Here's how the part is built. I have some questions about the finished solid (model axes, mm). A direction names the side the tool comes from. Round coordinates to 2 decimals unless told otherwise and drop trailing zeros. Write each loop counter-clockwise with the first axis right and the second up, starting at its lowest first coordinate (ties: lowest second). Pieces come first, ordered by that corner, then holes. Notation, with made-up numbers: (-38.75, 77.25) -> (15.25, 77.25) arc R16 ccw to (15.25, 99.25) -> close; hole circle Ø2 at (54, -14). An arc over 180 degrees is marked (long way). Answer in a Markdown table with one row per item.
from build123d import *

# Parameters (mm, degrees)
CROQUIS1_W                 = 56.1
CROQUIS1_H                 = 26.6
CROQUIS1_R                 = 2.1
CROQUIS1_W_2               = 40.9
CROQUIS1_H_2               = 20.6
SALIENTE_EXTRUIR1_DEPTH    = 8
CROQUIS2_W                 = 50.6
CROQUIS2_H                 = 26.6
SALIENTE_EXTRUIR2_DEPTH    = 8
CROQUIS3_W                 = 60.73602496
CROQUIS3_H                 = 26.6
SALIENTE_EXTRUIR3_DEPTH    = 8
CROQUIS4_R                 = 11.25
CORTAR_EXTRUIR1_DEPTH      = 5.5
CROQUIS5_R                 = 5.1
CORTAR_EXTRUIR2_DEPTH      = 62.563808362
CROQUIS6_R                 = 12.05
CROQUIS6_R_2               = 11.05
SALIENTE_EXTRUIR4_DEPTH    = 0.3
CHAFL_N1_SIZE              = 0.3
REDONDEO1_R                = 0.15
CHAFL_N2_SIZE              = 5
CORTAR_EXTRUIR5_REACH      = 65.536
CROQUIS11_W                = 30.047801794
CROQUIS11_H                = 26.6
CROQUIS12_R                = 1.45
CORTAR_EXTRUIR6_DEPTH      = 62.821699265
CHAFL_N8_SIZE              = 3
CHAFL_N9_SIZE              = 1
CHAFL_N10_SIZE             = 1.5
SALIENTE_EXTRUIR7_DEPTH    = 3
REDONDEO3_R                = 5
CROQUIS14_R                = 1.45
CORTAR_EXTRUIR7_DEPTH      = 70.085008007
CORTAR_EXTRUIR8_DEPTH      = 70.085008007
CORTAR_EXTRUIR8_DEPTH_BACK = 70.085008007
CROQUIS15_R                = 1.45


with BuildPart() as part:
    # Croquis1 → Saliente-Extruir1 (new body)
    with BuildSketch(Plane.XY):
        Rectangle(CROQUIS1_W, CROQUIS1_H)
        with Locations((24.250000128, -5)):
            Circle(CROQUIS1_R, mode=Mode.SUBTRACT)
        with Locations((24.250000128, 5)):
            Circle(CROQUIS1_R, mode=Mode.SUBTRACT)
        with Locations((-24.249999872, -5)):
            Circle(CROQUIS1_R, mode=Mode.SUBTRACT)
        with Locations((-24.249999872, 5)):
            Circle(CROQUIS1_R, mode=Mode.SUBTRACT)
        Rectangle(CROQUIS1_W_2, CROQUIS1_H_2, mode=Mode.SUBTRACT)
    extrude(amount=SALIENTE_EXTRUIR1_DEPTH)

    # Croquis2 → Saliente-Extruir2 (add)
    with BuildSketch(Plane(origin=(28.05, 0, 0), x_dir=(0, 0, -1), z_dir=(1, 0, 0))):
        with Locations((17.3, 0)):
            Rectangle(CROQUIS2_W, CROQUIS2_H)
    extrude(amount=SALIENTE_EXTRUIR2_DEPTH)

    # Croquis3 → Saliente-Extruir3 (add)
    with BuildSketch(Plane(origin=(0, 0, -42.6), x_dir=(-1, 0, 0), z_dir=(0, 0, -1))):
        with Locations((-5.68198752, 0)):
            Rectangle(CROQUIS3_W, CROQUIS3_H)
    extrude(amount=-SALIENTE_EXTRUIR3_DEPTH)

    # Croquis4 → Cortar-Extruir1 (cut)
    with BuildSketch(Plane.XY.offset(-34.6)):
        with Locations((-10.53602496, 0)):
            Circle(CROQUIS4_R)
    extrude(amount=-CORTAR_EXTRUIR1_DEPTH, mode=Mode.SUBTRACT)

    # Croquis5 → Cortar-Extruir2 (cut, through all)
    with BuildSketch(Plane.XY.offset(-40.1)):
        with Locations((-10.53602496, 0)):
            Circle(CROQUIS5_R)
    extrude(amount=-CORTAR_EXTRUIR2_DEPTH, mode=Mode.SUBTRACT)

    # Croquis6 → Saliente-Extruir4 (add)
    with BuildSketch(Plane.XY.offset(-34.6)):
        with Locations((-10.53602496, 0)):
            Circle(CROQUIS6_R)
        with Locations((-10.53602496, 0)):
            Circle(CROQUIS6_R_2, mode=Mode.SUBTRACT)
    extrude(amount=SALIENTE_EXTRUIR4_DEPTH)

    # Chaflán1
    chafl_n1_edges = [part.edges().sort_by_distance(p)[0] for p in [
        (-22.58602496, 0, -34.6),
    ]]
    chamfer(chafl_n1_edges, length=CHAFL_N1_SIZE - 0.0001)  # a hair under: the kernel refuses the full size

    # Redondeo1
    redondeo1_edges = [part.edges().sort_by_distance(p)[0] for p in [
        (-21.58602496, 0, -34.6),
        (-21.58602496, 0, -34.3),
    ]]
    fillet(redondeo1_edges, radius=REDONDEO1_R - 0.0001)  # a hair under: the kernel refuses the full size

    # Chaflán2
    chafl_n2_edges = [part.edges().sort_by_distance(p)[0] for p in [
        (-24.68602496, -13.3, -38.6),
        (-24.68602496, 13.3, -38.6),
    ]]
    chamfer(chafl_n2_edges, length=CHAFL_N2_SIZE)

    # Croquis11 → Cortar-Extruir5 (cut, up to next)
    with BuildSketch(Plane.XY.offset(8), mode=Mode.PRIVATE) as cortar_extruir5_sk1:
        with Locations((-15.023900897, 0)):
            Rectangle(CROQUIS11_W, CROQUIS11_H)
    cortar_extruir5_tool1 = extrude(cortar_extruir5_sk1.sketch, amount=-CORTAR_EXTRUIR5_REACH, mode=Mode.PRIVATE) & part.part
    add(cortar_extruir5_tool1.solids().sort_by_distance((-15.023901, 0, 8))[0], mode=Mode.SUBTRACT)

    # Croquis12 → Cortar-Extruir6 (cut, through all)
    with BuildSketch(Plane(origin=(0, -13.3, 0), x_dir=(-1, 0, 0), z_dir=(0, -1, 0))):
        with Locations(Location((-4.5, -4, 0), (0, 0, 90))):
            Circle(CROQUIS12_R)
    extrude(amount=-CORTAR_EXTRUIR6_DEPTH, mode=Mode.SUBTRACT)

    # Chaflán8
    chafl_n8_edges = [part.edges().sort_by_distance(p)[0] for p in [
        (-24.68602496, 0, -42.6),
        (-22.18602496, -10.8, -42.6),
        (-22.18602496, 10.8, -42.6),
        (8.18198752, -13.3, -42.6),
        (8.18198752, 13.3, -42.6),
        (36.05, 0, -42.6),
    ]]
    chamfer(chafl_n8_edges, length=CHAFL_N8_SIZE)

    # Chaflán9
    chafl_n9_edges = [part.edges().sort_by_distance(p)[0] for p in [
        (-15.63602496, 0, -42.6),
    ]]
    chamfer(chafl_n9_edges, length=CHAFL_N9_SIZE)

    # Chaflán10
    chafl_n10_edges = [part.edges().sort_by_distance(p)[0] for p in [
        (18.025, -13.3, 8),
        (36.05, 0, 8),
        (18.025, 13.3, 8),
    ]]
    chamfer(chafl_n10_edges, length=CHAFL_N10_SIZE)

    # Croquis13 → Saliente-Extruir7 (add)
    with BuildSketch(Plane(origin=(0, 13.3, 0), x_dir=(1, 0, 0), z_dir=(0, 1, 0))):
        with BuildLine():
            Line((28.05, 8.144334064), (28.05, 0))
            Line((28.05, 0), (9, 0))
            add(Edge.make_bspline(
                [(9, 0), (24.941361066, 0.053648998), (28.05, 8.144334064)],
                knots=[0, 0, 0, 0.673633708, 0.673633708, 0.673633708], degree=2))
        make_face()
    saliente_extruir7 = extrude(amount=-SALIENTE_EXTRUIR7_DEPTH)

    # Simetría7: Saliente-Extruir7 across plane
    add(saliente_extruir7.mirror(Plane.ZX))

    # Redondeo3
    redondeo3_edges = [part.edges().sort_by_distance(p)[0] for p in [
        (28.05, 0, -34.6),
    ]]
    fillet(redondeo3_edges, radius=REDONDEO3_R)

    # Croquis14 → Cortar-Extruir7 (cut, through all)
    with BuildSketch(Plane.ZY.offset(-28.05)):
        with Locations((-15.372167032, -8.3)):
            Circle(CROQUIS14_R)
        with Locations((-25.372167032, -8.3)):
            Circle(CROQUIS14_R)
    cortar_extruir7 = extrude(amount=-CORTAR_EXTRUIR7_DEPTH, mode=Mode.SUBTRACT)

    # Simetría8: Cortar-Extruir7 across plane
    add(cortar_extruir7.mirror(Plane.ZX), mode=Mode.SUBTRACT)

    # Croquis15 → Cortar-Extruir8 (cut, two sides: drawn at the far end of the back side and taken through both)
    with BuildSketch(Plane.ZY.offset(-28.05).offset(-CORTAR_EXTRUIR8_DEPTH_BACK)):
        with Locations((-20.372167032, 0)):
            Circle(CROQUIS15_R)
        with Locations((-30.372167032, 0)):
            Circle(CROQUIS15_R)
    extrude(amount=CORTAR_EXTRUIR8_DEPTH + CORTAR_EXTRUIR8_DEPTH_BACK, mode=Mode.SUBTRACT)


solid = part.part
1) I need wall thicknesses on line 1 (Z direction, x = 31, y = 8.3); line 2 (Y direction, x = 24, z = 2); line 3 (X direction, y = -11.8, z = 4). Which ranges of each line are inside material? Lowest first, please. Write a range as [from, to].
Response:
| item | result |
|---|---|
| line 1 | z = [-42.6, -26.82], [-23.92, -16.82], [-13.92, 8] |
| line 2 | y = [-13.3, -7.09], [-2.91, 2.91], [7.09, 13.3] |
| line 3 | x = [0, 3.05], [5.95, 36.05] |
2) We'd pull the mould along Z, two halves only. Please class faces 1 (the face through (0, -12, 4)), 2 (the face through (8.6, -11.8, -41.1)), 3 (the face through (4, 12, 0)), 4 (the face through (31.99, 7.08, -14.59)): +Z half, -Z half, draft (parallel to the pull), parting line (faces both ways), or undercut.
Response:
| item | result |
|---|---|
| face 1 | draft |
| face 2 | -Z half |
| face 3 | undercut |
| face 4 | undercut |
3) I want a section at B-B, the plane x = 7. List the corners of the cut face in (y, z) for me, and give its area (3 significant figures).
Response:
| item | result |
|---|---|
| outline | (-13.3, -39.6) -> (-10.3, -42.6) -> (10.3, -42.6) -> (13.3, -39.6) -> (13.3, -34.6) -> (-13.3, -34.6) -> close; (-13.3, 0) -> (-10.3, 0) -> (-10.3, 8) -> (-11.8, 8) -> (-13.3, 6.5) -> close; (10.3, 0) -> (13.3, 0) -> (13.3, 6.5) -> (11.8, 8) -> (10.3, 8) -> close |
| area | 250 mm^2 |
4) For pin 1 (12 mm diameter, centred on x = -16.5, y = 6.5, fed in from +Z); pin 2 (3.5 mm diameter, centred on y = 11, z = 5, fed in from -X); pin 3 (8 mm diameter, centred on y = 1.5, z = -21.5, fed in from -X), each with a flat end and sliding along its axis, tell me the tip position at first contact or that it passes through.
Response:
| item | result |
|---|---|
| pin 1 | stops at z = -34.3 |
| pin 2 | stops at x = 0 |
| pin 3 | stops at x = 28.05 |
5) I want a section at D-D, the plane x = 30.5. List the corners of the cut face in (y, z) for me, and give its area (3 significant figures).
Response:
| item | result |
|---|---|
| outline | (-13.3, -39.6) -> (-10.3, -42.6) -> (10.3, -42.6) -> (13.3, -39.6) -> (13.3, 6.5) -> (11.8, 8) -> (-11.8, 8) -> (-13.3, 6.5) -> close; hole circle Ø2.9 at (-8.3, -25.37); hole circle Ø2.9 at (-8.3, -15.37); hole circle Ø2.9 at (0, -30.37); hole circle Ø2.9 at (0, -20.37); hole circle Ø2.9 at (8.3, -25.37); hole circle Ø2.9 at (8.3, -15.37) |
| area | 1,300 mm^2 |
6) Which directions (+Z, -Z, +X, -X, +Y, -Y) give clear straight access to the entire face, cutting with the end or side of a thin tool? Please do faces 5 (the face through (-24.686, 0, -37)), 6 (the face through (25.38, 6.77, 3.94)), 7 (the face through (20.45, 0, 4)).
Response:
| item | result |
|---|---|
| face 5 | +Z, -Z, -X, +Y, -Y |
| face 6 | +Z |
| face 7 | +Z, -X |
7) I want a section at C-C, the plane y = 0. Count the separate pieces of the cut face and the enclosed holes in it, and give its area (3 significant figures).
Response:
| item | result |
|---|---|
| separate pieces | 4 |
| enclosed holes | 0 |
| area | 686 mm^2 |
8) I want a section at A-A, the plane z = 4. List the corners of the cut face in (x, y) for me.
Response:
| item | result |
|---|---|
| outline | (0, -13.3) -> (3.05, -13.3) -> (3.05, -10.3) -> (0, -10.3) -> close; (0, 10.3) -> (3.05, 10.3) -> (3.05, 13.3) -> (0, 13.3) -> close; (5.95, -13.3) -> (36.05, -13.3) -> (36.05, 13.3) -> (5.95, 13.3) -> (5.95, 10.3) -> (20.45, 10.3) -> (20.45, -10.3) -> (5.95, -10.3) -> close; hole circle Ø4.2 at (24.25, -5); hole circle Ø4.2 at (24.25, 5) |
